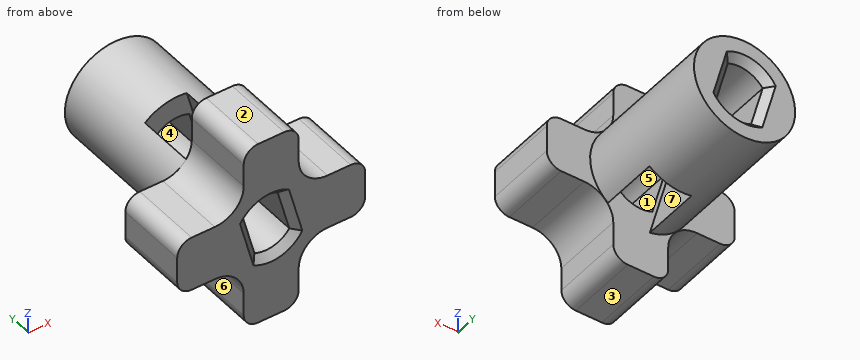
from build123d import *

# Parameters (mm, degrees)
SKETCH_1_R               = 3.5
EXTRUDE_1_DEPTH          = 15
EXTRUDE_2_DEPTH          = 5
CUT_EXTRUDE_1_DEPTH      = 15
CUT_EXTRUDE_2_DEPTH      = 15
CUT_EXTRUDE_2_DEPTH_BACK = 15
SKETCH_5_W               = 3
SKETCH_5_H               = 4
CHAMFER_1_SIZE           = 0.5


with BuildPart() as part:
    # Sketch 1 → Extrude 1 (new body)
    with BuildSketch(Plane(origin=(0, 0, 0), x_dir=(1, 0, 0), z_dir=(0, 1, 0))):
        with Locations(Location((0, 0, 0), (0, 0, 270))):
            Circle(SKETCH_1_R)
    extrude(amount=EXTRUDE_1_DEPTH)

    # Sketch 2 → Extrude 2 (add)
    with BuildSketch(Plane.XZ):
        with BuildLine():
            Line((0.9, 6.5), (-0.9, 6.5))
            ThreePointArc((-0.9, 6.5), (-1.607106781, 6.207106781), (-1.9, 5.5))
            Line((-1.9, 5.5), (-1.9, 3.9))
            ThreePointArc((-1.9, 3.9), (-2.485786438, 2.485786438), (-3.9, 1.9))
            Line((-3.9, 1.9), (-5.5, 1.9))
            ThreePointArc((-5.5, 1.9), (-6.207106781, 1.607106781), (-6.5, 0.9))
            Line((-6.5, 0.9), (-6.5, -0.9))
            ThreePointArc((-6.5, -0.9), (-6.207106781, -1.607106781), (-5.5, -1.9))
            Line((-5.5, -1.9), (-3.9, -1.9))
            ThreePointArc((-3.9, -1.9), (-2.485786438, -2.485786438), (-1.9, -3.9))
            Line((-1.9, -3.9), (-1.9, -5.5))
            ThreePointArc((-1.9, -5.5), (-1.607106781, -6.207106781), (-0.9, -6.5))
            Line((-0.9, -6.5), (0.9, -6.5))
            ThreePointArc((0.9, -6.5), (1.607106781, -6.207106781), (1.9, -5.5))
            Line((1.9, -5.5), (1.9, -3.9))
            ThreePointArc((1.9, -3.9), (2.485786438, -2.485786438), (3.9, -1.9))
            Line((3.9, -1.9), (5.5, -1.9))
            ThreePointArc((5.5, -1.9), (6.207106781, -1.607106781), (6.5, -0.9))
            Line((6.5, -0.9), (6.5, 0.9))
            ThreePointArc((6.5, 0.9), (6.207106781, 1.607106781), (5.5, 1.9))
            Line((5.5, 1.9), (3.9, 1.9))
            ThreePointArc((3.9, 1.9), (2.485786438, 2.485786438), (1.9, 3.9))
            Line((1.9, 3.9), (1.9, 5.5))
            ThreePointArc((1.9, 5.5), (1.607106781, 6.207106781), (0.9, 6.5))
        make_face()
    extrude(amount=-EXTRUDE_2_DEPTH)

    # Sketch 3 → Cut-Extrude 1 (cut)
    with BuildSketch(Plane(origin=(0, 15, 0), x_dir=(1, 0, 0), z_dir=(0, 1, 0))):
        with BuildLine():
            Line((1.207407283, -0.323523806), (0.803326178, -1.831575019))
            ThreePointArc((0.803326178, -1.831575019), (-0.51763809, -1.931851653), (-1.611488388, -1.184527407))
            Line((-1.611488388, -1.184527407), (-1.207407283, 0.323523806))
            Line((-1.207407283, 0.323523806), (-0.803326178, 1.831575019))
            ThreePointArc((-0.803326178, 1.831575019), (0.51763809, 1.931851653), (1.611488388, 1.184527407))
            Line((1.611488388, 1.184527407), (1.207407283, -0.323523806))
        make_face()
    extrude(amount=-CUT_EXTRUDE_1_DEPTH, mode=Mode.SUBTRACT)

    # Sketch 5 → Cut-Extrude 2 (cut, two sides: drawn at the far end of the back side and taken through both)
    with BuildSketch(Plane(origin=(0, 0, 0), x_dir=(-0.96592582628907, 0, -0.2588190451025146), z_dir=(0.2588190451025146, 0, -0.96592582628907)).offset(-CUT_EXTRUDE_2_DEPTH_BACK)):
        with Locations((0, 7)):
            Rectangle(SKETCH_5_W, SKETCH_5_H)
    extrude(amount=CUT_EXTRUDE_2_DEPTH + CUT_EXTRUDE_2_DEPTH_BACK, mode=Mode.SUBTRACT)

    # Chamfer 1
    chamfer_1_edges = [part.edges().sort_by_distance(p)[0] for p in [
        (1.207407283, 0, 0.323523806),
        (-0.51763809, 0, 1.931851653),
        (-1.207407283, 0, -0.323523806),
        (0.51763809, 0, -1.931851653),
        (1.207407283, 15, 0.323523806),
        (0.51763809, 15, -1.931851653),
        (-1.207407283, 15, -0.323523806),
        (-0.51763809, 15, 1.931851653),
    ]]
    chamfer(chamfer_1_edges, length=CHAMFER_1_SIZE)


solid = part.part
Work out the finished part from the listing and answer in its coordinate system (mm). Face numbers are marked on the shaded views. A direction names the side the tool comes from. Give positions to 0.01 mm unless a question says otherwise; leave off trailing zeros. Order: outer loops, then holes, each group sorted by start corner. A loop starts at its lowest first (then second) coordinate and runs counter-clockwise, first axis right, second up. Notation, with made-up numbers: (4, 23.25) -> (48, 23.25) arc R28 ccw to (48, 51.25) -> close; hole circle Ø7 at (31.5, 26). An arc over 180 degrees is marked (long way). One line per item, written item: value.
Item 1: Find section A-A, the plane x = 0. Give the vertices of the cut face in (y, z).
Answer sheet:
outline: (0, -6.5) -> (5, -6.5) -> (5, -2) -> (0.5, -2) -> (0, -2.5) -> close; (0, 2.5) -> (0.5, 2) -> (5, 2) -> (5, 6.5) -> (0, 6.5) -> close; (9, -3.5) -> (15, -3.5) -> (15, -2.5) -> (14.5, -2) -> (9, -2) -> close; (9, 2) -> (14.5, 2) -> (15, 2.5) -> (15, 3.5) -> (9, 3.5) -> close
Item 2: Find section D-D, the plane y = 10. Give the vertices of the cut face in (x, z), plus the area to 3 significant figures.
Answer sheet:
outline: circle Ø7 at (0, 0); hole (-1.61, 1.18) -> (-0.8, -1.83) arc R2 ccw to (1.61, -1.18) -> (0.8, 1.83) arc R2 ccw to start
area: 29.2 mm²
Item 3: Find section B-B, the plane z = 0. Give the vertices of the cut face in (x, y).
Answer sheet:
outline: (-6.5, 0) -> (-1.81, 0) -> (-1.29, 0.5) -> (-1.29, 5) -> (-1.55, 5) -> (-1.55, 9) -> (-1.29, 9) -> (-1.29, 14.5) -> (-1.81, 15) -> (-3.5, 15) -> (-3.5, 5) -> (-6.5, 5) -> close; (1.29, 0.5) -> (1.81, 0) -> (6.5, 0) -> (6.5, 5) -> (3.5, 5) -> (3.5, 15) -> (1.81, 15) -> (1.29, 14.5) -> (1.29, 9) -> (1.55, 9) -> (1.55, 5) -> (1.29, 5) -> close
Item 4: Find section C-C, the plane y = 8. Give the vertices of the cut face in (x, z).
Answer sheet:
outline: (-2.27, 2.67) arc R3.5 ccw to (-0.63, -3.44) -> close; (0.63, 3.44) -> (2.27, -2.67) arc R3.5 ccw to start
Item 5: A tool of negligible diameter and unlimited length cuts with its end or side. For the marked faces 5, 6 and 7, from which of +Z, -Z, +X, -X, +Y, -Y can it reach the whole face along a straight path? Write none if from no direction.
Answer sheet:
face 5: +Y, -Y
face 6: -Z, -X, +Y, -Y
face 7: +Z
Item 6: Determine the mould class of the marked faces 1, 2, 3 and 4 for opening direction Z: released by +Z, released by -Z, zero draft, split by the parting line, or undercut.
Answer sheet:
face 1: undercut
face 2: released by +Z
face 3: released by -Z
face 4: undercut
Item 7: Straight lines are drawn through the part: probe 1 along X at (y, z) = (11.25, 0.75); probe 2 along Y at (x, z) = (-0.5, 3.5); probe 3 along X at (y, z) = (8.5, 0.25). For each, find the intervals that lie inside material, in ascending order.
Answer sheet:
probe 1: -3.42 to -1.5, 1.09 to 3.42
probe 2: 0 to 5
probe 3: -3.49 to -1.62, 1.49 to 3.49
Item 8: Flat-ended cylindrical pins translate along their axes: P1, Ø1.8, axis at x = 5, y = 2.5, coming from the -Z side; P2, Ø0.8, axis at y = 1.5, z = 4.5, coming from the -X side; P3, Ø5, axis at y = 10, z = -2, coming from the -X side. Find the tip coordinate at first contact, or state that the pin passes through.
Answer sheet:
P1: z = -1.9
P2: x = -1.9
P3: x = -3.5
